```python
from build123d import *

# Parameters (mm, degrees)
SKETCH1_W           = 95.25
SKETCH1_H           = 41.91
BOSS_EXTRUDE1_DEPTH = 1.5875
SKETCH2_R           = 14.224
SKETCH2_R_2         = 2.286
SKETCH2_R_3         = 2.032
CUT_EXTRUDE1_DEPTH  = 3.175


with BuildPart() as part:
    # Sketch1 → Boss-Extrude1 (new, symmetric)
    with BuildSketch(Plane.XY):
        with Locations((-2.54, -2.667)):
            Rectangle(SKETCH1_W, SKETCH1_H)
    extrude(amount=BOSS_EXTRUDE1_DEPTH, both=True)

    # Sketch2 → Cut-Extrude1 (cut)
    with BuildSketch(Plane(origin=(0, 0, -1.5875), x_dir=(-1, 0, 0), z_dir=(0, 0, -1))):
        with Locations((2.413, -3.048)):
            Circle(SKETCH2_R)
        with Locations((-15.260103904, -20.364606719)):
            Circle(SKETCH2_R_2)
        with Locations((-15.260103904, 15.195393281)):
            Circle(SKETCH2_R_3)
        with Locations((20.299896096, 15.195393281)):
            Circle(SKETCH2_R_2)
        with Locations((20.299896096, -20.364606719)):
            Circle(SKETCH2_R_3)
    extrude(amount=-CUT_EXTRUDE1_DEPTH, mode=Mode.SUBTRACT)


solid = part.part
```
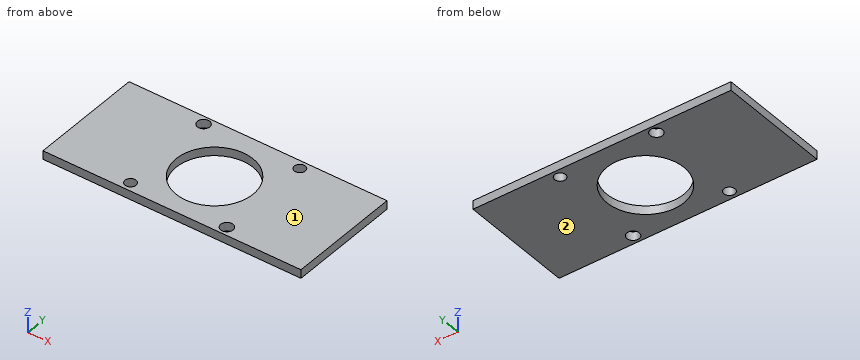
Could you check a few things on this model? Use its own coordinates, in mm. Face numbers are marked on the shaded views. Give positions to 0.01 mm unless a question says otherwise; leave off trailing zeros. Write each loop counter-clockwise with the first axis right and the second up, starting at its lowest first coordinate (ties: lowest second). Pieces come first, ordered by that corner, then holes. Notation, with made-up numbers: (18, 70.25) -> (58, 70.25) arc R18 cw to (58, 91.25) -> close; hole circle Ø9 at (87, 80.25). An arc over 180 degrees is marked (long way). Write each question's results on one line, items separated by ' | '.
1. I want a section at B-B, the plane x = -11.5. Write out the boundary of the cut face in (y, z).
Check sheet entries:
outline: (-23.62, -1.59) -> (-13.99, -1.59) -> (-13.99, 1.59) -> (-23.62, 1.59) -> close; (7.89, -1.59) -> (18.29, -1.59) -> (18.29, 1.59) -> (7.89, 1.59) -> close
2. I need wall thicknesses on L1, parallel to Y at x = -20, z = 0.55; L2, parallel to X at y = 9, z = 0.4 (3 decimals); L3, parallel to Y at x = -15.5, z = -0.95. Which ranges of each line are inside material? Lowest first, please.
Check sheet entries:
L1: y = -23.62 to -22.37, -18.35 to 12.93, 17.46 to 18.29 | L2: x = -50.165 to -9.974, 5.148 to 45.085 | L3: y = -23.62 to -8.62, 2.52 to 18.29
3. I want a section at A-A, the plane y = -10.5. Write out the boundary of the cut face in (x, z) (1 decimal), then the cut area to 3 significant figures.
Check sheet entries:
outline: (-50.2, -1.6) -> (-14.5, -1.6) -> (-14.5, 1.6) -> (-50.2, 1.6) -> close; (9.7, -1.6) -> (45.1, -1.6) -> (45.1, 1.6) -> (9.7, 1.6) -> close | area: 225 mm²
4. I want a section at D-D, the plane z = 0.6. Write out the boundary of the cut face in (x, y) (3 decimals).
Check sheet entries:
outline: (-50.165, -23.622) -> (45.085, -23.622) -> (45.085, 18.288) -> (-50.165, 18.288) -> close; hole circle Ø4.572 at (-20.3, 15.195); hole circle Ø4.064 at (-20.3, -20.365); hole circle Ø28.448 at (-2.413, -3.048); hole circle Ø4.572 at (15.26, -20.365); hole circle Ø4.064 at (15.26, 15.195)
5. If we mould it in two halves opening along Z, with no side actions, what happens to the marked faces 1 and 2? For each: released by +Z, released by -Z, zero draft, split by the parting line, or undercut.
Check sheet entries:
face 1: released by +Z | face 2: released by -Z
6. I want a section at C-C, the plane y = 14. Write out the boundary of the cut face in (x, z) (1 decimal).
Check sheet entries:
outline: (-50.2, -1.6) -> (-22.2, -1.6) -> (-22.2, 1.6) -> (-50.2, 1.6) -> close; (-18.4, -1.6) -> (13.6, -1.6) -> (13.6, 1.6) -> (-18.4, 1.6) -> close; (16.9, -1.6) -> (45.1, -1.6) -> (45.1, 1.6) -> (16.9, 1.6) -> close
